from build123d import *

# Parameters (mm, degrees)
SKETCH1_R               = 40
BOSS_EXTRUDE1_DEPTH     = 6
SKETCH2_R               = 17
BOSS_EXTRUDE2_DEPTH     = 3
CUT_EXTRUDE1_DEPTH      = 58.280013966
CUT_EXTRUDE1_DEPTH_BACK = 58.280013966
SKETCH3_R               = 6.25
SKETCH3_R_2             = 2.15


with BuildPart() as part:
    # Sketch1 → Boss-Extrude1 (new body)
    with BuildSketch(Plane.XY):
        Circle(SKETCH1_R)
    extrude(amount=BOSS_EXTRUDE1_DEPTH)

    # Sketch2 → Boss-Extrude2 (add)
    with BuildSketch(Plane.XY.offset(6)):
        Circle(SKETCH2_R)
    extrude(amount=BOSS_EXTRUDE2_DEPTH)

    # Sketch3 → Cut-Extrude1 (cut, two sides: drawn at the far end of the back side and taken through both)
    with BuildSketch(Plane.XY.offset(9).offset(-CUT_EXTRUDE1_DEPTH_BACK)):
        Circle(SKETCH3_R)
        with Locations((0, 12.5)):
            Circle(SKETCH3_R_2)
        with Locations((12.5, 0)):
            Circle(SKETCH3_R_2)
        with Locations((0, -12.5)):
            Circle(SKETCH3_R_2)
        with Locations((-12.5, 0)):
            Circle(SKETCH3_R_2)
    extrude(amount=CUT_EXTRUDE1_DEPTH + CUT_EXTRUDE1_DEPTH_BACK, mode=Mode.SUBTRACT)


solid = part.part
Could you check a few things on this model? Use its own coordinates, in mm. A direction names the side the tool comes from. Coordinates: 2 decimals unless noted, no trailing zeros. Write each loop counter-clockwise with the first axis right and the second up, starting at its lowest first coordinate (ties: lowest second). Pieces come first, ordered by that corner, then holes. Notation, with made-up numbers: (6, 35.5) - (28, 35.5) arc R27 cw to (28, 74.5) - close; hole circle Ø7 at (52, -24.5). An arc over 180 degrees is marked (long way). Put each result on its own line as item: value. Start each with the question number.
Q1. I want a section at B-B on z = 1.25. Write out the boundary of the cut face in (x, y), plus the area to 3 significant figures.
Q2. I want a section at C-C on y = 12.5. Write out the boundary of the cut face in (x, z), plus the area to 3 significant figures.
Q3. Thinking about a two-plate mould opening in Y: for faces 1 (the flat face through (-0.6, -17.2, 6)), 2 (the cylindrical face through (-8.67, -39.05, 2.96)), 3 (the cylindrical face through (-10.45, 0.65, 4.44)), which applies, pulls with the +Y half, pulls with the -Y half, needs draft (parallel to the pull), parting line crosses it, or undercut?
Q4. I'm going to push flat-ended pins straight in: P1, Ø4, axis at x = 21, z = 2.5, coming from the -Y side; P2, Ø4, axis at y = 16, z = 5, coming from the +X side; P3, Ø1.5, axis at y = 15, z = 2.5, coming from the -X side. Where does each tip first touch, or does it pass through?
Q5. I want a section at A-A on x = 0. Write out the boundary of the cut face in (y, z), plus the area to 3 significant figures.
Q6. I want a section at D-D on y = -16. Write out the boundary of the cut face in (x, z), plus the area to 3 significant figures.
Q7. Which directions (+Z, -Z, +X, -X, +Y, -Y) give clear straight access to the entire face, cutting with the end or side of a thin tool? Please do faces 4 (the cylindrical face through (9.139, 14.334, 7.479)), 5 (the cylindrical face through (-1.706, 11.192, 4.437)).
Q8. Please list where these lines run through material, in increasing order: L1, parallel to Y at x = 0, z = 2.5; L2, parallel to Z at x = 24.5, y = 24; L3, parallel to X at y = -12.5, z = 3.25.
Checks:
1. outline: circle Ø80 at (0, 0); hole circle Ø4.3 at (-12.5, 0); hole circle Ø12.5 at (0, 0); hole circle Ø4.3 at (0, -12.5); hole circle Ø4.3 at (0, 12.5); hole circle Ø4.3 at (12.5, 0)
1. area: 4,850 mm²
2. outline: (-38, 0) - (-2.15, 0) - (-2.15, 9) - (-11.52, 9) - (-11.52, 6) - (-38, 6) - close; (2.15, 0) - (38, 0) - (38, 6) - (11.52, 6) - (11.52, 9) - (2.15, 9) - close
2. area: 486 mm²
3. face 1: needs draft
3. face 2: parting line crosses it
3. face 3: undercut
4. P1: y = -35.2
4. P2: x = 37.47
4. P3: x = -37.38
5. outline: (-40, 0) - (-14.65, 0) - (-14.65, 9) - (-17, 9) - (-17, 6) - (-40, 6) - close; (-10.35, 0) - (-6.25, 0) - (-6.25, 9) - (-10.35, 9) - close; (6.25, 0) - (10.35, 0) - (10.35, 9) - (6.25, 9) - close; (14.65, 0) - (40, 0) - (40, 6) - (17, 6) - (17, 9) - (14.65, 9) - close
5. area: 392 mm²
6. outline: (-36.66, 0) - (36.66, 0) - (36.66, 6) - (5.74, 6) - (5.74, 9) - (-5.74, 9) - (-5.74, 6) - (-36.66, 6) - close
6. area: 474 mm²
7. face 4: +Z
7. face 5: +Z, -Z
8. L1: -40 to -14.65, -10.35 to -6.25, 6.25 to 10.35, 14.65 to 40
8. L2: 0 to 6
8. L3: -38 to -2.15, 2.15 to 38
